from build123d import *

# Parameters (mm, degrees)
CYLINDER1538_R     = 1.5
CYLINDER1538_DEPTH = 100
CYLINDER1537_R     = 1.5
CYLINDER1537_DEPTH = 100
CYLINDER1532_R     = 1.5
CYLINDER1532_DEPTH = 32
CYLINDER1531_R     = 1.5
CYLINDER1531_DEPTH = 32
BOX520_W           = 200
BOX520_H           = 100
BOX520_DEPTH       = 100
BOX518_W           = 200
BOX518_H           = 100
BOX518_DEPTH       = 100
CYLINDER1127_R     = 4
CYLINDER1127_DEPTH = 100
CYLINDER1128_R     = 4
CYLINDER1128_DEPTH = 100
CYLINDER1129_R     = 4
CYLINDER1129_DEPTH = 100
CYLINDER1125_R     = 4
CYLINDER1125_DEPTH = 100
CYLINDER1130_R     = 4
CYLINDER1130_DEPTH = 100
CYLINDER1126_R     = 4
CYLINDER1126_DEPTH = 100
CYLINDER1492_R     = 1.5
CYLINDER1492_DEPTH = 100
CYLINDER1493_R     = 1.5
CYLINDER1493_DEPTH = 100
CYLINDER1494_R     = 1.5
CYLINDER1494_DEPTH = 100
CYLINDER1495_R     = 1.5
CYLINDER1495_DEPTH = 100
CYLINDER1496_R     = 1.5
CYLINDER1496_DEPTH = 100
CYLINDER1497_R     = 1.5
CYLINDER1497_DEPTH = 100
CYLINDER1498_R     = 1.5
CYLINDER1498_DEPTH = 100
CYLINDER1491_R     = 1.5
CYLINDER1491_DEPTH = 100
CYLINDER1490_R     = 59
CYLINDER1490_DEPTH = 4


with BuildPart() as obj1:
    # Cylinder1538 → Cylinder1538 (new body)
    with BuildSketch(Plane(origin=(14, 0, -60), x_dir=(1, 0, 0), z_dir=(0, 0, 1))):
        Circle(CYLINDER1538_R)
    extrude(amount=CYLINDER1538_DEPTH)


with BuildPart() as obj2:
    # Cylinder1537 → Cylinder1537 (new body)
    with BuildSketch(Plane(origin=(90, 0, -60), x_dir=(1, 0, 0), z_dir=(0, 0, 1))):
        Circle(CYLINDER1537_R)
    extrude(amount=CYLINDER1537_DEPTH)

    # Compound889: union obj1
    add(obj1.part)


with BuildPart() as obj3:
    # Cylinder1532 → Cylinder1532 (new body)
    with BuildSketch(Plane(origin=(78, 41, -42), x_dir=(1, 0, 0), z_dir=(0, 0, 1))):
        Circle(CYLINDER1532_R)
    extrude(amount=CYLINDER1532_DEPTH)


with BuildPart() as compound901:
    # Cylinder1531 → Cylinder1531 (new body)
    with BuildSketch(Plane(origin=(26, 41, -42), x_dir=(1, 0, 0), z_dir=(0, 0, 1))):
        Circle(CYLINDER1531_R)
    extrude(amount=CYLINDER1531_DEPTH)

    # Compound901: union obj3
    add(obj3.part)


with BuildPart() as krychle520:
    # Box520 → Box520 (new body)
    with BuildSketch(Plane(origin=(-60, 44, -90), x_dir=(1, 0, 0), z_dir=(0, 0, 1))):
        with Locations((100, 50)):
            Rectangle(BOX520_W, BOX520_H)
    extrude(amount=BOX520_DEPTH)


with BuildPart() as krychle518:
    # Box518 → Box518 (new body)
    with BuildSketch(Plane(origin=(-60, -124, -90), x_dir=(1, 0, 0), z_dir=(0, 0, 1))):
        with Locations((100, 50)):
            Rectangle(BOX518_W, BOX518_H)
    extrude(amount=BOX518_DEPTH)


with BuildPart() as obj4:
    # Cylinder1127 → Cylinder1127 (new body)
    with BuildSketch(Plane(origin=(-36, 34, -90), x_dir=(1, 0, 0), z_dir=(0, 0, 1))):
        Circle(CYLINDER1127_R)
    extrude(amount=CYLINDER1127_DEPTH)


with BuildPart() as obj5:
    # Cylinder1128 → Cylinder1128 (new body)
    with BuildSketch(Plane(origin=(-36, -34, -90), x_dir=(1, 0, 0), z_dir=(0, 0, 1))):
        Circle(CYLINDER1128_R)
    extrude(amount=CYLINDER1128_DEPTH)


with BuildPart() as obj6:
    # Cylinder1129 → Cylinder1129 (new body)
    with BuildSketch(Plane(origin=(50, 0, -90), x_dir=(1, 0, 0), z_dir=(0, 0, 1))):
        Circle(CYLINDER1129_R)
    extrude(amount=CYLINDER1129_DEPTH)


with BuildPart() as obj7:
    # Cylinder1125 → Cylinder1125 (new body)
    with BuildSketch(Plane(origin=(36, 34, -90), x_dir=(1, 0, 0), z_dir=(0, 0, 1))):
        Circle(CYLINDER1125_R)
    extrude(amount=CYLINDER1125_DEPTH)


with BuildPart() as obj8:
    # Cylinder1130 → Cylinder1130 (new body)
    with BuildSketch(Plane(origin=(36, -34, -90), x_dir=(1, 0, 0), z_dir=(0, 0, 1))):
        Circle(CYLINDER1130_R)
    extrude(amount=CYLINDER1130_DEPTH)


with BuildPart() as obj9:
    # Cylinder1126 → Cylinder1126 (new body)
    with BuildSketch(Plane(origin=(-50, 0, -90), x_dir=(1, 0, 0), z_dir=(0, 0, 1))):
        Circle(CYLINDER1126_R)
    extrude(amount=CYLINDER1126_DEPTH)

    # Compound896: union obj4, obj5, obj6, obj7, obj8
    add(obj4.part)
    add(obj5.part)
    add(obj6.part)
    add(obj7.part)
    add(obj8.part)


with BuildPart() as obj10:
    # Cylinder1492 → Cylinder1492 (new body)
    with BuildSketch(Plane(origin=(103, 6, -60), x_dir=(1, 0, 0), z_dir=(0, 0, 1))):
        Circle(CYLINDER1492_R)
    extrude(amount=CYLINDER1492_DEPTH)


with BuildPart() as obj11:
    # Cylinder1493 → Cylinder1493 (new body)
    with BuildSketch(Plane(origin=(76, 18, -60), x_dir=(1, 0, 0), z_dir=(0, 0, 1))):
        Circle(CYLINDER1493_R)
    extrude(amount=CYLINDER1493_DEPTH)


with BuildPart() as obj12:
    # Cylinder1494 → Cylinder1494 (new body)
    with BuildSketch(Plane(origin=(91, -21, -60), x_dir=(1, 0, 0), z_dir=(0, 0, 1))):
        Circle(CYLINDER1494_R)
    extrude(amount=CYLINDER1494_DEPTH)


with BuildPart() as obj13:
    # Cylinder1495 → Cylinder1495 (new body)
    with BuildSketch(Plane(origin=(13, -21, -60), x_dir=(1, 0, 0), z_dir=(0, 0, 1))):
        Circle(CYLINDER1495_R)
    extrude(amount=CYLINDER1495_DEPTH)


with BuildPart() as obj14:
    # Cylinder1496 → Cylinder1496 (new body)
    with BuildSketch(Plane(origin=(28, 18, -60), x_dir=(1, 0, 0), z_dir=(0, 0, 1))):
        Circle(CYLINDER1496_R)
    extrude(amount=CYLINDER1496_DEPTH)


with BuildPart() as obj15:
    # Cylinder1497 → Cylinder1497 (new body)
    with BuildSketch(Plane(origin=(1, -12, -60), x_dir=(1, 0, 0), z_dir=(0, 0, 1))):
        Circle(CYLINDER1497_R)
    extrude(amount=CYLINDER1497_DEPTH)


with BuildPart() as obj16:
    # Cylinder1498 → Cylinder1498 (new body)
    with BuildSketch(Plane(origin=(1, 6, -60), x_dir=(1, 0, 0), z_dir=(0, 0, 1))):
        Circle(CYLINDER1498_R)
    extrude(amount=CYLINDER1498_DEPTH)


with BuildPart() as obj17:
    # Cylinder1491 → Cylinder1491 (new body)
    with BuildSketch(Plane(origin=(103, -12, -60), x_dir=(1, 0, 0), z_dir=(0, 0, 1))):
        Circle(CYLINDER1491_R)
    extrude(amount=CYLINDER1491_DEPTH)

    # Compound893: union obj10, obj11, obj12, obj13, obj14, obj15, obj16
    add(obj10.part)
    add(obj11.part)
    add(obj12.part)
    add(obj13.part)
    add(obj14.part)
    add(obj15.part)
    add(obj16.part)


with BuildPart() as cut526:
    # Cylinder1490 → Cylinder1490 (new body)
    with BuildSketch(Plane(origin=(52, 0, -26), x_dir=(1, 0, 0), z_dir=(0, 0, 1))):
        Circle(CYLINDER1490_R)
    extrude(amount=CYLINDER1490_DEPTH)

    # Cut513: cut obj17
    add(obj17.part, mode=Mode.SUBTRACT)

    # Cut514: cut obj9
    add(obj9.part, mode=Mode.SUBTRACT)

    # Cut520: cut Krychle518
    add(krychle518.part, mode=Mode.SUBTRACT)

    # Cut522: cut Krychle520
    add(krychle520.part, mode=Mode.SUBTRACT)

    # Cut523: cut Compound901
    add(compound901.part, mode=Mode.SUBTRACT)

    # Cut526: cut obj2
    add(obj2.part, mode=Mode.SUBTRACT)


solid = cut526.part
Could you check a few things on this model? Use its own coordinates, in mm. Give positions to 0.01 mm unless a question says otherwise; leave off trailing zeros. Write each loop counter-clockwise with the first axis right and the second up, starting at its lowest first coordinate (ties: lowest second). Pieces come first, ordered by that corner, then holes. Notation, with made-up numbers: (6, 78) - (20, 78) arc R25 cw to (20, 109) - close; hole circle Ø9 at (54, 50.25). An arc over 180 degrees is marked (long way). Use CSV: the item, a comma, the result in double quotes. Start each with the question number.
Item 1: If I drill on line 1 along X through (y, z) = (0, -23.7); line 2 along Y through (x, z) = (78, -23); line 3 along X through (y, z) = (6, -23.75), over which ranges is the centre line in solid material (lowest first)?
Item 2: I want a section at B-B, the plane x = 36. Please give me the cut outline in (y, z).
Item 3: If we mould it in two halves opening along Y, with no side actions, what happens to faces 1 (the face through (2.386, 5.425, -24.028)), 2 (the face through (51, 44, -24)), 3 (the face through (51, 10, -22))? For each: pulls with the +Y half, pulls with the -Y half, needs draft (parallel to the pull), parting line crosses it, or undercut.
Item 4: I want a section at A-A, the plane y = 0. Please give me the cut outline in (x, z).
Item 5: I'm going to push flat-ended pins straight in: pin 1 (1.5 mm diameter, centred on y = 32.5, z = -24, fed in from -X); pin 2 (1.5 mm diameter, centred on y = 26.5, z = -23.5, fed in from -X); pin 3 (1.5 mm diameter, centred on y = 7, z = -24, fed in from +X). Where does each tip first touch, or does it pass through?
Item 6: I want a section at C-C, the plane z = -23.6. Give the number of separate pieces and of enclosed holes in the cut face, then the cut area to 3 significant figures.
Item 7: I want a section at D-D, the plane y = 41. Please give me the cut outline in (x, z).
Findings:
1,line 1,"x = -7 to 12.5, 15.5 to 46, 54 to 88.5, 91.5 to 111"
1,line 2,"y = -24 to 39.5, 42.5 to 44"
1,line 3,"x = -6.69 to -0.5, 2.5 to 101.5, 104.5 to 110.69"
2,outline,"(-24, -26) - (30, -26) - (30, -22) - (-24, -22) - close; (38, -26) - (44, -26) - (44, -22) - (38, -22) - close"
3,face 1,"undercut"
3,face 2,"pulls with the +Y half"
3,face 3,"needs draft"
4,outline,"(-7, -26) - (12.5, -26) - (12.5, -22) - (-7, -22) - close; (15.5, -26) - (46, -26) - (46, -22) - (15.5, -22) - close; (54, -26) - (88.5, -26) - (88.5, -22) - (54, -22) - close; (91.5, -26) - (111, -26) - (111, -22) - (91.5, -22) - close"
5,pin 1,"stops at x = 2.27"
5,pin 2,"stops at x = -1.08"
5,pin 3,"stops at x = 110.67"
6,separate pieces,"1"
6,enclosed holes,"14"
6,area,"7,230 mm2"
7,outline,"(9.57, -26) - (24.5, -26) - (24.5, -22) - (9.57, -22) - close; (27.5, -26) - (76.5, -26) - (76.5, -22) - (27.5, -22) - close; (79.5, -26) - (94.43, -26) - (94.43, -22) - (79.5, -22) - close"
